Could you check a few things on this model? Use its own coordinates, in mm. Round coordinates to 2 decimals unless told otherwise and drop trailing zeros. Write each loop counter-clockwise with the first axis right and the second up, starting at its lowest first coordinate (ties: lowest second). Pieces come first, ordered by that corner, then holes. Notation, with made-up numbers: (21, 5.5) -> (60, 5.5) arc R30 cw to (60, 40.5) -> close; hole circle Ø9 at (25.5, -9.5). An arc over 180 degrees is marked (long way). Answer as CSV lines item,"result". Start each with the question number.
Q1. Imagine slicing it at A-A on y = 15. Please give me the cut outline in (x, z).
Q2. If I drill on line 1 (X direction, y = 32.5, z = 0.55); line 2 (Y direction, x = 5.5, z = -0.6); line 3 (Z direction, x = 5.25, y = 28), over which ranges is the centre line in solid material (lowest first)? Write a range as [from, to].
Q3. Will these pins go through, and if not, where does the flat tip stop? pin 1 Ø4 at (x, y) = (3.5, 13) entering from +Z; pin 2 Ø1.5 at (x, y) = (2.5, 17) entering from -Z.
Q4. Imagine slicing it at B-B on x = 4. Please give me the cut outline in (y, z), and give its area (3 significant figures).
Q5. If we mould it in two halves opening along Y, with no side actions, what happens to faces 1 (the cylindrical face through (6.8, 26.7, -0.6)), 2 (the cylindrical face through (5.603, 9.472, 0.052)), 3 (the flat face through (6, 41.937, 0)), 4 (the conical face through (1.37, 0.23, -0.07))? For each: pulls with the +Y half, pulls with the -Y half, needs draft (parallel to the pull), parting line crosses it, or undercut.
from build123d import *

# Parameters (mm, degrees)
SKETCH2_R               = 0.5
CUT_EXTRUDE1_DEPTH      = 4.052867504
CUT_EXTRUDE1_DEPTH_BACK = 4.052867504
SKETCH3_R               = 0.4
SKETCH5_R               = 1
BOSS_EXTRUDE1_DEPTH     = 30


with BuildPart() as part:
    # Sketch1 → Revolve1 (revolve)
    with BuildSketch(Plane.XY, mode=Mode.PRIVATE) as revolve1_sk:
        Polygon((0, 0), (3, 0), (3, -0.4), (2.268512728, -0.4), align=None)
    revolve(revolve1_sk.sketch.rotate(Axis((0, 0, 0), (-1, 0, 0)), 180), axis=Axis((0, 0, 0), (-1, 0, 0)))

    # Sketch2 → Cut-Extrude1 (cut, two sides)
    with BuildSketch(Plane(origin=(0, 0, 0), x_dir=(1, 0, 0), z_dir=(0, 1, 0))) as cut_extrude1_sk:
        Circle(SKETCH2_R)
    extrude(amount=CUT_EXTRUDE1_DEPTH, mode=Mode.SUBTRACT)
    extrude(cut_extrude1_sk.sketch, amount=-CUT_EXTRUDE1_DEPTH_BACK, mode=Mode.SUBTRACT)

    # Sweep1: sweep along a path in Sketch4
    with BuildLine(Plane.XY) as sweep1_path:
        Line((3, 0), (4.483768236, 0))
        ThreePointArc((4.483768236, 0), (6.592246851, 1.156750979), (6.749537704, 3.556545654))
        ThreePointArc((6.749537704, 3.556545654), (6.189631943, 5.205974837), (6, 6.937491748))
        Line((6, 6.937491748), (6, 11.937491748))
    # Sketch3 → Sweep1 (sweep)
    with BuildSketch(Plane(origin=(3, 0, 0), x_dir=(0, 0, -1), z_dir=(1, 0, 0))):
        Circle(SKETCH3_R)
    sweep(path=sweep1_path.line)

    # Sketch5 → Boss-Extrude1 (add)
    with BuildSketch(Plane(origin=(0, 11.937491748, 0), x_dir=(-1, 0, 0), z_dir=(0, 1, 0))):
        with Locations((-6, 0)):
            Circle(SKETCH5_R)
    extrude(amount=BOSS_EXTRUDE1_DEPTH)


solid = part.part
Checks:
1,outline,"circle Ø2 at (6, 0)"
2,line 1,"[5.16, 6.84]"
2,line 2,"[11.94, 41.94]"
2,line 3,"[-0.66, 0.66]"
3,pin 1,"z = 0.87"
3,pin 2,"through"
4,outline,"circle Ø0.8 at (0, 0)"
4,area,"0.503 mm^2"
5,face 1,"needs draft"
5,face 2,"undercut"
5,face 3,"pulls with the +Y half"
5,face 4,"parting line crosses it"
